Read the model definition and answer for the solid it produces. Units are mm, in the model's axes. Give positions to 0.01 mm unless a question says otherwise; leave off trailing zeros. Write each loop counter-clockwise with the first axis right and the second up, starting at its lowest first coordinate (ties: lowest second). Pieces come first, ordered by that corner, then holes. Notation, with made-up numbers: M 0.25,-22.5 L 9.25,-22.5 A4 ccw 9.25,-16.5 Z; hole C 15.25,82 d6. An arc over 180 degrees is marked long. Answer as CSV lines item,"result". Start each with the question number.
```python
from build123d import *


with BuildPart() as f1:
    # F0 (on Front) → F1 (revolve)
    with BuildSketch(Plane.XZ):
        with BuildLine():
            Line((-47, 0), (-25, 0))
            Line((-25, 0), (-25, 2.153316))
            ThreePointArc((-25, 2.153316), (-25.540882, 3.45912), (-26.846686, 4.000002))
            Line((-26.846686, 4.000002), (-36, 2))
            Line((-36, 2), (-45.153314, 3.999998))
            ThreePointArc((-45.153314, 3.999998), (-46.459118, 3.459117), (-47, 2.153313))
            Line((-47, 2.153313), (-47, 0))
        make_face()
    revolve(axis=Axis((0, 0, 2), (0, 0, 1)))


solid = f1.part
```
1. Find section C-C on z = 1. Determine the outline of the cut face in (x, y), then the cut area to 3 significant figures.
2. Given pin 1 (10 mm diameter, centred on x = 0, y = 15, fed in from +Z); pin 2 (1.5 mm diameter, centred on y = -29, z = 3, fed in from -X), each flat-ended and moving along its own axis, determine where each tip first touches the part or whether it passes through.
3. Find section A-A on y = 0. Determine the outline of the cut face in (x, z), then the cut area to 3 significant figures.
4. Determine the mould class of faces 1 (the face through (-44.83, -14.12, 1.06)), 2 (the face through (-20, 20, 0)), 3 (the face through (7.928, 35.703, 2.125)) for opening direction Y: +Y half, -Y half, draft (parallel to the pull), parting line (faces both ways), or undercut.
5. Find the intervals of material crossed by line 1 (Y direction, x = 0, z = 1.2); line 2 (X direction, y = -3, z = 1.35), in increasing order. Write a range as [from, to].
Computed:
1,outline,"C 0,0 d94; hole C 0,0 d50"
1,area,"4,980 mm^2"
2,pin 1,"passes through"
2,pin 2,"stops at x = -37.41"
3,outline,"M -47,0 L -25,0 L -25,2.15 A1.85 ccw -26.85,4 L -36,2 L -45.15,4 A1.85 ccw -47,2.15 Z; M 25,0 L 47,0 L 47,2.15 A1.85 ccw 45.15,4 L 36,2 L 26.85,4 A1.85 ccw 25,2.15 Z"
3,area,"136 mm^2"
4,face 1,"parting line"
4,face 2,"draft"
4,face 3,"undercut"
5,line 1,"y = [-47, -25], [25, 47]"
5,line 2,"x = [-46.9, -24.82], [24.82, 46.9]"
